```python
from build123d import *

# Parameters (mm, degrees)
SKETCH_1_W             = 40
SKETCH_1_H             = 50
SKETCH_1_R             = 2
SM_BASE_FLANGE_1_DEPTH = 3
SM_EDGE_FLANGE_1_DEPTH = 50
SKETCH_12_R            = 4
CUT_EXTRUDE_1_DEPTH    = 75.006756448


# Sheet-metal steps are written as plain solids
with BuildPart() as part:
    # Sketch 1 → 基体-法兰1 (new body)
    with BuildSketch(Plane(origin=(0, 0, 0), x_dir=(1, 0, 0), z_dir=(0, 1, 0))):
        Rectangle(SKETCH_1_W, SKETCH_1_H)
        with Locations(Location((12.1, 15, 0), (0, 0, 270))):
            Circle(SKETCH_1_R, mode=Mode.SUBTRACT)
        with Locations(Location((-12.1, -15, 0), (0, 0, 270))):
            Circle(SKETCH_1_R, mode=Mode.SUBTRACT)
        with Locations(Location((-12.1, 15, 0), (0, 0, 270))):
            Circle(SKETCH_1_R, mode=Mode.SUBTRACT)
        with Locations(Location((12.1, -15, 0), (0, 0, 270))):
            Circle(SKETCH_1_R, mode=Mode.SUBTRACT)
    extrude(amount=-SM_BASE_FLANGE_1_DEPTH)

    # 边线-法兰1 section (across the edge) → 边线-法兰1 (add)
    with BuildSketch(Plane(origin=(-21, -3, 25), x_dir=(1, 0, 0), z_dir=(0, 0, -1))):
        with BuildLine():
            Line((-3, 1), (-3, 51))
            Line((-3, 51), (0, 51))
            Line((0, 51), (0, 1))
            ThreePointArc((0, 1), (0.292893219, 0.292893219), (1, 0))
            Line((1, 0), (1, -3))
            ThreePointArc((1, -3), (-1.828427125, -1.828427125), (-3, 1))
        make_face()
    extrude(amount=SM_EDGE_FLANGE_1_DEPTH)

    # 草图12 → 切除-拉伸1 (cut, through all)
    with BuildSketch(Plane.ZY.offset(24)):
        with Locations(Location((0, -29, 0), (0, 0, 270))):
            Circle(SKETCH_12_R)
    extrude(amount=-CUT_EXTRUDE_1_DEPTH, mode=Mode.SUBTRACT)


solid = part.part
```
Here's how the part is built. I have some questions about the finished solid (model axes, mm). A direction names the side the tool comes from. Round coordinates to 2 decimals unless told otherwise and drop trailing zeros. Order: outer loops, then holes, each group sorted by start corner. A loop starts at its lowest first (then second) coordinate and runs counter-clockwise, first axis right, second up. Notation, with made-up numbers: (70.5, -28.5) -> (97.5, -28.5) arc R28 ccw to (97.5, 0.5) -> close; hole circle Ø6 at (75.25, 38.5). An arc over 180 degrees is marked (long way). Use a Markdown table: item, result. Add a question column.
(1) Suppose I cut it at A-A, the plane z = 0. Please give me the cut outline in (x, y), and give its area (3 significant figures).
(2) Suppose I cut it at B-B, the plane x = -12.1. Please give me the cut outline in (y, z), and give its area (3 significant figures).
(3) I need wall thicknesses on line 1 along Z through (x, y) = (-12, -2); line 2 along Z through (x, y) = (-23.1, -29); line 3 along X through (y, z) = (-1.7, -15). Which ranges of each line are inside material? Lowest first, please.
(4) If we mould it in two halves opening along Z, with no side actions, what happens to faces 3 (the face through (14.083, -1.479, -15.26)), 4 (the face through (-23, -54, 0)), 5 (the face through (-21.5, -19.1, 25))? For each: released by +Z, released by -Z, zero draft, split by the parting line, or undercut.
(5) Suppose I cut it at C-C, the plane y = -29. Please give me the cut outline in (x, z).
(6) Suppose I cut it at D-D, the plane z = -15. Please give me the cut outline in (x, y), and give its area (3 significant figures).
(7) For pin 1 Ø12 at (y, z) = (-37.5, -17.5) entering from +X; pin 2 Ø7 at (y, z) = (-29, 0) entering from -X; pin 3 Ø6 at (x, z) = (-1, 19.5) entering from -Y, each with a flat end and sliding along its axis, tell me the tip position at first contact or that it passes through.
(8) For faces 1 (the face through (-21, -35, 0)), 2 (the face through (-14.052, -1.479, 14.566)), which set-ups out of +Z, -Z, +X, -X, +Y, -Y let a thin tool reach every point of the face, with its end or its side?
Verdict:
| question | item | result |
|---|---|---|
| 1 | outline | (-24, -54) -> (-21, -54) -> (-21, -33) -> (-24, -33) -> close; (-24, -25) -> (-21, -25) -> (-21, -4) arc R1 cw to (-20, -3) -> (20, -3) -> (20, 0) -> (-20, 0) arc R4 ccw to (-24, -4) -> close |
| 1 | area | 258 mm2 |
| 2 | outline | (-3, -25) -> (0, -25) -> (0, -17) -> (-3, -17) -> close; (-3, -13) -> (0, -13) -> (0, 13) -> (-3, 13) -> close; (-3, 17) -> (0, 17) -> (0, 25) -> (-3, 25) -> close |
| 2 | area | 126 mm2 |
| 3 | line 1 | -25 to -17, -13 to 13, 17 to 25 |
| 3 | line 2 | -25 to -4, 4 to 25 |
| 3 | line 3 | -23.27 to -14.1, -10.1 to 10.1, 14.1 to 20 |
| 4 | face 3 | undercut |
| 4 | face 4 | zero draft |
| 4 | face 5 | released by +Z |
| 5 | outline | (-24, -25) -> (-21, -25) -> (-21, -4) -> (-24, -4) -> close; (-24, 4) -> (-21, 4) -> (-21, 25) -> (-24, 25) -> close |
| 6 | outline | (-24, -54) -> (-21, -54) -> (-21, -4) arc R1 cw to (-20, -3) -> (-14.1, -3) -> (-14.1, 0) -> (-20, 0) arc R4 ccw to (-24, -4) -> close; (-10.1, -3) -> (10.1, -3) -> (10.1, 0) -> (-10.1, 0) -> close; (14.1, -3) -> (20, -3) -> (20, 0) -> (14.1, 0) -> close |
| 6 | area | 258 mm2 |
| 7 | pin 1 | x = -21 |
| 7 | pin 2 | through |
| 7 | pin 3 | y = -3 |
| 8 | face 1 | +Z, -Z, +X, -Y |
| 8 | face 2 | +Y, -Y |
